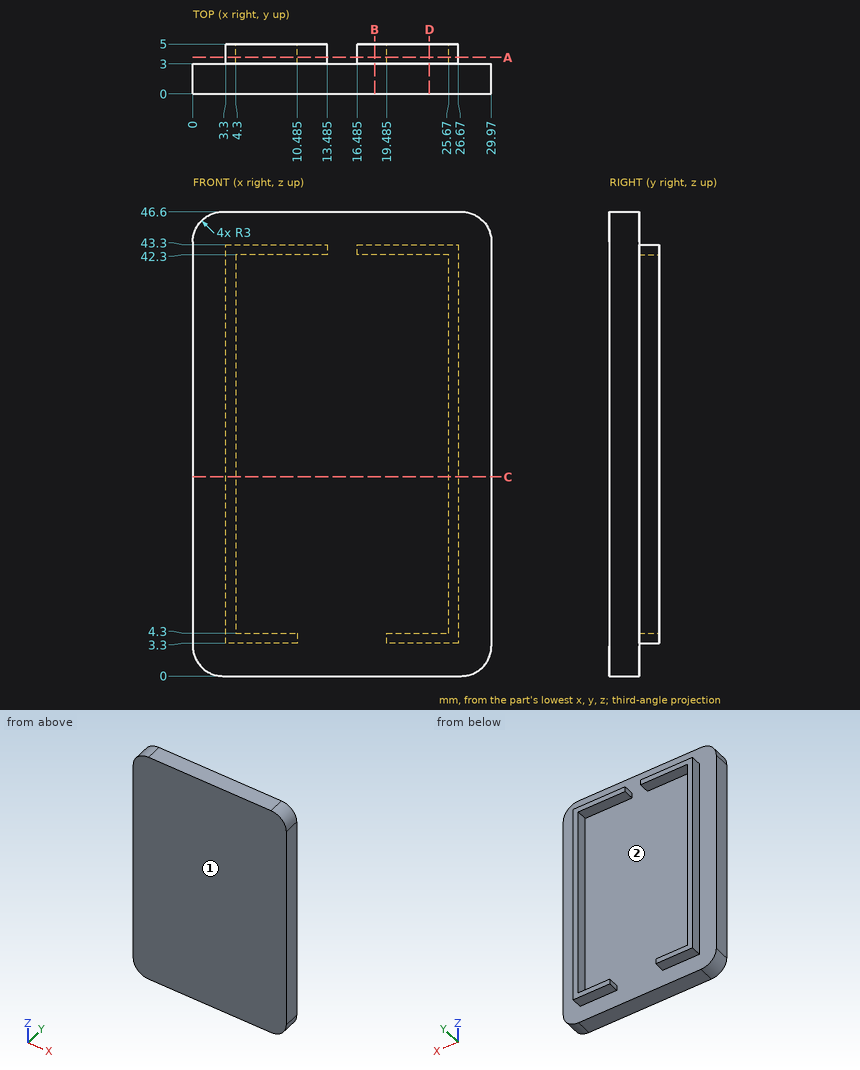
Design review of the part shown in the three views and the two pictorial views. Dimensions are in mm from the part's minimum x, y and z. Round coordinates to 2 decimals unless told otherwise and drop trailing zeros. Order: outer loops, then holes, each group sorted by start corner. A loop starts at its lowest first (then second) coordinate and runs counter-clockwise, first axis right, second up.
(1) Take a section at B-B, the plane x = 18.25. State the section outline as (y, z) points, plus the area to 3 significant figures.
Working result:
outline: (0, 0) - (3, 0) - (3, 42.3) - (5, 42.3) - (5, 43.3) - (3, 43.3) - (3, 46.6) - (0, 46.6) - close
area: 142 mm2
(2) Take a section at D-D, the plane x = 23.75. State the section outline as (y, z) points.
Working result:
outline: (0, 0) - (3, 0) - (3, 3.3) - (5, 3.3) - (5, 4.3) - (3, 4.3) - (3, 42.3) - (5, 42.3) - (5, 43.3) - (3, 43.3) - (3, 46.6) - (0, 46.6) - close
(3) For P1, Ø0.8, axis at y = 4, z = 43, coming from the +X side; P2, Ø0.6, axis at x = 22.5, y = 4.5, coming from the +Z side; P3, Ø1, axis at x = 24, y = 4, coming from the -Z side, all flat-tipped, find the tip position at first contact; note any pin that passes through.
Working result:
P1: stops at x = 26.67
P2: stops at z = 43.3
P3: stops at z = 3.3
(4) Take a section at C-C, the plane z = 20. State the section outline as (x, y) points.
Working result:
outline: (0, 0) - (29.97, 0) - (29.97, 3) - (26.67, 3) - (26.67, 5) - (25.67, 5) - (25.67, 3) - (4.3, 3) - (4.3, 5) - (3.3, 5) - (3.3, 3) - (0, 3) - close
(5) Wall thickness on L1, parallel to X at y = 3.15, z = 17; L2, parallel to Z at x = 8.5, y = 3.2; L3, parallel to Y at x = 6, z = 30: over which ranges is each line inside the solid? List them lowest first.
Working result:
L1: x = 3.3 to 4.3, 25.67 to 26.67
L2: z = 3.3 to 4.3, 42.3 to 43.3
L3: y = 0 to 3
(6) Take a section at A-A, the plane y = 3.65. State the section outline as (x, z) points (3 decimals), plus the area to 3 significant figures.
Working result:
outline: (3.3, 3.3) - (10.485, 3.3) - (10.485, 4.3) - (4.3, 4.3) - (4.3, 42.3) - (13.485, 42.3) - (13.485, 43.3) - (3.3, 43.3) - close; (16.485, 42.3) - (25.67, 42.3) - (25.67, 4.3) - (19.485, 4.3) - (19.485, 3.3) - (26.67, 3.3) - (26.67, 43.3) - (16.485, 43.3) - close
area: 111 mm2
(7) Mouldability with a two-part tool opening along Z and no side actions: class the marked faces 1 and 2 as released by +Z, released by -Z, zero draft, split by the parting line, or undercut.
Working result:
face 1: zero draft
face 2: undercut
